For this review, take the finished solid that the model builds, in its own axes (mm). A direction names the side the tool comes from. Coordinates: 2 decimals unless noted, no trailing zeros. Order: outer loops, then holes, each group sorted by start corner. A loop starts at its lowest first (then second) coordinate and runs counter-clockwise, first axis right, second up. Notation, with made-up numbers: (-24, -27) -> (13, -27) arc R31 ccw to (13, 5) -> close; hole circle Ø5 at (8.25, 4). An arc over 180 degrees is marked (long way). Return JSON: item names as keys, results as strings. Group by question number.
Item 1: Draft analysis for pull direction X (two halves, no side actions). For faces 4 (the cylindrical face through (-15.945, -15.745, -29.324)), 5 (the flat face through (0, -31.75, 29)), state which applies: +X half, -X half, draft (parallel to the pull), parting line (faces both ways), or undercut.
Item 2: For line 1 along Z through (x, y) = (10, 5.5); line 2 along Z through (x, y) = (17, 22); line 3 along Y through (x, z) = (-9, 27.5), list the stretches that pass through material, from the lowest coordinate up.
Item 3: Insertion check: pin 1 (13 mm diameter, centred on y = 32, z = -8.5, fed in from -X); pin 2 (13 mm diameter, centred on y = 32, z = 6, fed in from -X); pin 3 (4 mm diameter, centred on x = -8.5, z = 3, fed in from -Y); pin 4 (3 mm diameter, centred on x = -8.5, z = 23.5, fed in from +Y). Each pin has a flat end and moves straight along its axis. Give the tip position at first contact, or say it passes through.
Item 4: Take a section at B-B (y = -14). Write out the cut boundary in (x, z).
Item 5: Take a section at C-C (y = 29). Write out the cut boundary in (x, z) (3 decimals), then the cut area to 3 significant figures.
Item 6: Take a section at D-D (x = 14.5). Write out the cut boundary in (y, z), then the cut area to 3 significant figures.
Item 7: Machinability: for faces 1 (the flat face through (-12.7, -23, 29)), 2 (the flat face through (0, -16, 26.194)), 3 (the cylindrical face through (-15.841, 3.219, -25.045)), which of the approach directions +Z, -Z, +X, -X, +Y, -Y give a long, thin tool a straight path to every point of the face, cutting with its end or side? Answer none if there is none.
Item 8: Take a section at A-A (z = -2). Count the separate pieces of the cut face and the enclosed holes in it, then the cut area to 3 significant figures.
```python
from build123d import *

# Parameters (mm, degrees)
SKETCH1_W           = 50.8
SKETCH1_H           = 65.0875
BOSS_EXTRUDE1_DEPTH = 6.35
SKETCH2_W           = 50.8
SKETCH2_H           = 6.35
BOSS_EXTRUDE2_DEPTH = 31.75
SKETCH4_W           = 25.233918668
SKETCH4_H           = 33.3375
CUT_EXTRUDE1_DEPTH  = 31.75
SKETCH5_W           = 31.75
SKETCH5_H           = 42.8625
BOSS_EXTRUDE3_DEPTH = 49.53
SKETCH4_2_W         = 25.233918668
SKETCH4_2_H         = 33.3375
CUT_EXTRUDE2_DEPTH  = 58.7375
CUT_EXTRUDE4_DEPTH  = 58.7375
SKETCH8_W           = 26.9875
SKETCH8_H           = 38.1
CUT_EXTRUDE7_DEPTH  = 58.7375
SKETCH12_W          = 3.208041114
SKETCH12_H          = 30.1625
CUT_EXTRUDE13_DEPTH = 12.7
CUT_EXTRUDE14_DEPTH = 76.2
CUT_EXTRUDE15_DEPTH = 76.2
CUT_EXTRUDE16_DEPTH = 76.2


with BuildPart() as part:
    # Sketch1 → Boss-Extrude1 (new body)
    with BuildSketch(Plane(origin=(0, 0, 0), x_dir=(1, 0, 0), z_dir=(0, 1, 0))):
        Rectangle(SKETCH1_W, SKETCH1_H)
    extrude(amount=BOSS_EXTRUDE1_DEPTH)

    # Sketch2 → Boss-Extrude2 (add)
    with BuildSketch(Plane(origin=(0, 0, 0), x_dir=(-1, 0, 0), z_dir=(0, -1, 0))):
        with Locations((0, -29.36875)):
            Rectangle(SKETCH2_W, SKETCH2_H)
        with Locations((0, 29.36875)):
            Rectangle(SKETCH2_W, SKETCH2_H)
    extrude(amount=BOSS_EXTRUDE2_DEPTH)

    # Sketch4 → Cut-Extrude1 (cut)
    with BuildSketch(Plane(origin=(0, 6.35, 0), x_dir=(1, 0, 0), z_dir=(0, 1, 0))):
        with Locations((9.608040666, 0)):
            Rectangle(SKETCH4_W, SKETCH4_H)
    extrude(amount=-CUT_EXTRUDE1_DEPTH, mode=Mode.SUBTRACT)

    # Sketch5 → Boss-Extrude3 (add)
    with BuildSketch(Plane(origin=(0, 6.35, 0), x_dir=(1, 0, 0), z_dir=(0, 1, 0))):
        with Locations((9.525, 0)):
            Rectangle(SKETCH5_W, SKETCH5_H)
    extrude(amount=BOSS_EXTRUDE3_DEPTH)

    # Sketch4<2> → Cut-Extrude2 (cut)
    with BuildSketch(Plane(origin=(0, 6.35, 0), x_dir=(1, 0, 0), z_dir=(0, 1, 0))):
        with Locations((9.608040666, 0)):
            Rectangle(SKETCH4_2_W, SKETCH4_2_H)
    extrude(amount=CUT_EXTRUDE2_DEPTH, mode=Mode.SUBTRACT)

    # Sketch7 → Cut-Extrude4 (cut)
    with BuildSketch(Plane.XY.offset(21.43125)):
        with BuildLine():
            Line((19.05, 25.7175), (19.05, 51.1175))
            ThreePointArc((19.05, 51.1175), (20.6375, 52.705), (22.225, 51.1175))
            Line((22.225, 51.1175), (22.225, 25.7175))
            ThreePointArc((22.225, 25.7175), (20.6375, 24.13), (19.05, 25.7175))
        make_face()
        with BuildLine():
            Line((0, 51.1175), (0, 25.7175))
            ThreePointArc((0, 25.7175), (-1.5875, 24.13), (-3.175, 25.7175))
            Line((-3.175, 25.7175), (-3.175, 51.1175))
            ThreePointArc((-3.175, 51.1175), (-1.5875, 52.705), (0, 51.1175))
        make_face()
    extrude(amount=-CUT_EXTRUDE4_DEPTH, mode=Mode.SUBTRACT)

    # Sketch8 → Cut-Extrude7 (cut)
    with BuildSketch(Plane(origin=(25.4, 0, 0), x_dir=(0, 0, -1), z_dir=(1, 0, 0))):
        with Locations((0, 25.4)):
            Rectangle(SKETCH8_W, SKETCH8_H)
    extrude(amount=-CUT_EXTRUDE7_DEPTH, mode=Mode.SUBTRACT)

    # Sketch12 → Cut-Extrude13 (cut)
    with BuildSketch(Plane(origin=(0, 0, 0), x_dir=(-1, 0, 0), z_dir=(0, -1, 0))):
        with Locations((4.612939225, 1.5875)):
            Rectangle(SKETCH12_W, SKETCH12_H)
    extrude(amount=-CUT_EXTRUDE13_DEPTH, mode=Mode.SUBTRACT)

    # Sketch14 → Cut-Extrude14 (cut)
    with BuildSketch(Plane.XY.offset(32.54375)):
        with BuildLine():
            Line((12.7, -18.919342158), (12.7, -26.800657842))
            ThreePointArc((12.7, -26.800657842), (9.525, -29.975657842), (6.35, -26.800657842))
            Line((6.35, -26.800657842), (6.35, -18.919342158))
            ThreePointArc((6.35, -18.919342158), (9.525, -15.744342158), (12.7, -18.919342158))
        make_face()
        with BuildLine():
            Line((-12.7, -18.919342158), (-12.7, -26.800657842))
            ThreePointArc((-12.7, -26.800657842), (-15.875, -29.975657842), (-19.05, -26.800657842))
            Line((-19.05, -26.800657842), (-19.05, -18.919342158))
            ThreePointArc((-19.05, -18.919342158), (-15.875, -15.744342158), (-12.7, -18.919342158))
        make_face()
    extrude(amount=-CUT_EXTRUDE14_DEPTH, mode=Mode.SUBTRACT)

    # Sketch15 → Cut-Extrude15 (cut)
    with BuildSketch(Plane.XY.offset(32.54375)):
        with BuildLine():
            Line((-11.481562965, -1.962227272), (12.734603348, -1.962227272))
            ThreePointArc((12.734603348, -1.962227272), (16.958353287, -6.18597721), (12.734603348, -10.409727149))
            Line((12.734603348, -10.409727149), (-11.481562965, -10.409727149))
            ThreePointArc((-11.481562965, -10.409727149), (-15.705312903, -6.18597721), (-11.481562965, -1.962227272))
        make_face()
    extrude(amount=-CUT_EXTRUDE15_DEPTH, mode=Mode.SUBTRACT)

    # Sketch16 → Cut-Extrude16 (cut)
    with BuildSketch(Plane(origin=(0, 6.35, 0), x_dir=(1, 0, 0), z_dir=(0, 1, 0))):
        with BuildLine():
            Line((-9.797813027, 19.133291295), (-9.797813027, -19.133291295))
            ThreePointArc((-9.797813027, -19.133291295), (-15.71106294, -25.046541209), (-21.624312854, -19.133291295))
            Line((-21.624312854, -19.133291295), (-21.624312854, 19.133291295))
            ThreePointArc((-21.624312854, 19.133291295), (-15.71106294, 25.046541209), (-9.797813027, 19.133291295))
        make_face()
    extrude(amount=-CUT_EXTRUDE16_DEPTH, mode=Mode.SUBTRACT)


solid = part.part
```
Findings below:
{
 "1": {"face 4": "undercut", "face 5": "draft"},
 "2": {"line 1": "z = -32.54 to -16.67, 16.67 to 32.54", "line 2": "z = -21.43 to -16.67, 16.67 to 21.43", "line 3": "y = -31.75 to -10.41, -1.96 to 6.35"},
 "3": {"pin 1": "stops at x = -6.35", "pin 2": "passes through", "pin 3": "stops at y = 0", "pin 4": "stops at y = 6.35"},
 "4": {"outline": "(-25.4, -32.54) -> (25.4, -32.54) -> (25.4, -26.19) -> (-25.4, -26.19) -> close; (-25.4, 26.19) -> (25.4, 26.19) -> (25.4, 32.54) -> (-25.4, 32.54) -> close"},
 "5": {"outline": "(-6.35, -21.431) -> (-3.175, -21.431) -> (-3.175, -13.494) -> (-6.35, -13.494) -> close; (-6.35, 13.494) -> (-3.175, 13.494) -> (-3.175, 21.431) -> (-6.35, 21.431) -> close; (0, -21.431) -> (19.05, -21.431) -> (19.05, -16.669) -> (0, -16.669) -> close; (0, 16.669) -> (19.05, 16.669) -> (19.05, 21.431) -> (0, 21.431) -> close; (22.225, -21.431) -> (25.4, -21.431) -> (25.4, -13.494) -> (22.225, -13.494) -> close; (22.225, 13.494) -> (25.4, 13.494) -> (25.4, 21.431) -> (22.225, 21.431) -> close", "area": "282 mm2"},
 "6": {"outline": "(-31.75, -32.54) -> (-10.02, -32.54) -> (-10.02, -26.19) -> (-31.75, -26.19) -> close; (-31.75, 26.19) -> (-10.02, 26.19) -> (-10.02, 32.54) -> (-31.75, 32.54) -> close; (-2.35, -32.54) -> (6.35, -32.54) -> (6.35, -21.43) -> (55.88, -21.43) -> (55.88, -16.67) -> (0, -16.67) -> (0, -26.19) -> (-2.35, -26.19) -> close; (-2.35, 26.19) -> (0, 26.19) -> (0, 16.67) -> (55.88, 16.67) -> (55.88, 21.43) -> (6.35, 21.43) -> (6.35, 32.54) -> (-2.35, 32.54) -> close", "area": "979 mm2"},
 "7": {"face 1": "+Z, -Z", "face 2": "+X, -X, -Y", "face 3": "+Y, -Y"},
 "8": {"separate pieces": "5", "enclosed holes": "0", "area": "140 mm2"}
}
